Source: CAD feature listing. Evaluate the final solid. Frame: model axes, mm. A direction names the side the tool comes from. Give positions to 0.01 mm unless a question says otherwise; leave off trailing zeros. Order: outer loops, then holes, each group sorted by start corner. A loop starts at its lowest first (then second) coordinate and runs counter-clockwise, first axis right, second up. Notation, with made-up numbers: M -2,45 L 10,45 A31 cw 10,80 Z; hole C -10.5,-39.5 d10. An arc over 180 degrees is marked long. Answer in a Markdown table with one row per item. Add a question column.
(1) Section query C-C, the plane y = 8.5. Return loops of the section in (x, z), plus the area to 3 significant figures.
(2) Section query D-D, the plane x = -35. Return loops of the section in (y, z), plus the area to 3 significant figures.
(3) Mould query, pull axis Y, two halves, no side actions, for faces 1 (the face through (110.507, 6.458, 22.745)), 2 (the face through (44, 0, 0)), 3 (the face through (24, 30, 10)), 4 (the face through (-53, 0, 10)). Classes: pulls with the +Y half, pulls with the -Y half, needs draft (parallel to the pull), parting line crosses it, or undercut.
(4) Pin query (flat end, axial travel): P1, Ø5, axis at x = -48, y = -9, coming from the +Z side; P2, Ø9, axis at x = -48, y = 0, coming from the -Z side; P3, Ø1, axis at y = 16.5, z = 12, coming from the -X side; P4, Ø6.5, axis at y = -28, z = 13.5, coming from the +X side. Return the tip coordinate at first contact, or that it passes through.
(5) Material intervals for line 1 along Y through (x, z) = (0, 13); line 2 along Z through (x, y) = (-25.5, 19); line 3 along Y through (x, z) = (74.5, 28), sorted ascending.
(6) Section query B-B, the plane z = 12.5. Count the separate pieces of the cut face and the enclosed holes in it, plus the area to 3 significant figures.
(7) Section query A-A, the plane x = 0. Return loops of the section in (y, z), plus the area to 3 significant figures.
(8) Set-up query: faces 5 (the face through (90, 0, 5)), 6 (the face through (70, 9, 40)), 7 (the face through (90, -27, 10)), 8 (the face through (90, 27, 10)). Return all of +Z, -Z, +X, -X, +Y, -Y with unobstructed straight access to the full face (end or side cutting, diameter ignored); none if empty.
from build123d import *
from build123d.topology import SkipClean

# Parameters (mm, degrees)
SKETCH1_R           = 30
BOSS_EXTRUDE1_DEPTH = 20
SKETCH2_R           = 27.5
CUT_EXTRUDE1_DEPTH  = 47.904157598
BOSS_EXTRUDE2_START = -20
BOSS_EXTRUDE2_DEPTH = 20
SKETCH6_R           = 21.5
CUT_EXTRUDE2_DEPTH  = 35
SKETCH11_R          = 24
BOSS_EXTRUDE3_DEPTH = 20
BOSS_EXTRUDE4_START = -40
SKETCH12_R          = 24
BOSS_EXTRUDE4_DEPTH = 40
SKETCH13_R          = 21.5
CUT_EXTRUDE6_DEPTH  = 35
BOSS_EXTRUDE6_START = -20
BOSS_EXTRUDE6_DEPTH = 20
SKETCH15_R          = 5
CUT_EXTRUDE8_DEPTH  = 20
FILLET1_R           = 30
FILLET2_R           = 30


with BuildPart() as part:
    # Sketch1 → Boss-Extrude1 (new body)
    with BuildSketch(Plane.XY):
        Circle(SKETCH1_R)
    extrude(amount=BOSS_EXTRUDE1_DEPTH)

    # Sketch2 → Cut-Extrude1 (cut, through all)
    with BuildSketch(Plane.XY.offset(20)):
        Circle(SKETCH2_R)
    extrude(amount=-CUT_EXTRUDE1_DEPTH, mode=Mode.SUBTRACT)

    # Sketch4 → Boss-Extrude2 (add)
    with BuildSketch(Plane.XY.offset(20).offset(BOSS_EXTRUDE2_START)):
        with BuildLine():
            Line((0, 30), (90, 30))
            Line((90, 30), (90, 24))
            ThreePointArc((90, 24), (114, 0), (90, -24))
            Line((90, -24), (90, -30))
            Line((90, -30), (0, -30))
            ThreePointArc((0, -30), (30, 0), (0, 30))
        make_face()
    extrude(amount=BOSS_EXTRUDE2_DEPTH)

    # Sketch6 → Cut-Extrude2 (cut)
    with BuildSketch(Plane.XY.offset(20)):
        with Locations((90, 0)):
            Circle(SKETCH6_R)
    extrude(amount=-CUT_EXTRUDE2_DEPTH, mode=Mode.SUBTRACT)

    # Sketch11 → Boss-Extrude3 (add)
    with SkipClean():  # the faces are left unmerged after this step: merging them gives an invalid solid
        with BuildSketch(Plane.XY.offset(20)):
            with Locations((90, 0)):
                Circle(SKETCH11_R)
        extrude(amount=BOSS_EXTRUDE3_DEPTH)
    add(part.part.scale(1), mode=Mode.REPLACE)  # the faces are merged on a copy

    # Sketch12 → Boss-Extrude4 (add)
    with SkipClean():  # the faces are left unmerged after this step: merging them gives an invalid solid
        with BuildSketch(Plane.XY.offset(40).offset(BOSS_EXTRUDE4_START)):
            with Locations((90, 0)):
                Circle(SKETCH12_R)
        extrude(amount=BOSS_EXTRUDE4_DEPTH)

    # Sketch13 → Cut-Extrude6 (cut)
    with SkipClean():  # the faces are left unmerged after this step: merging them gives an invalid solid
        with BuildSketch(Plane.XY.offset(40)):
            with Locations((90, 0)):
                Circle(SKETCH13_R)
        extrude(amount=-CUT_EXTRUDE6_DEPTH, mode=Mode.SUBTRACT)

    # Sketch14 → Boss-Extrude6 (add)
    with BuildSketch(Plane.XY.offset(20).offset(BOSS_EXTRUDE6_START)):
        with BuildLine():
            ThreePointArc((0, 30), (-30, 0), (0, -30))
            Line((0, -30), (-69.770044623, -30))
            Line((-69.770044623, -30), (-69.770044623, 30))
            Line((-69.770044623, 30), (0, 30))
        make_face()
    extrude(amount=BOSS_EXTRUDE6_DEPTH)

    # Sketch15 → Cut-Extrude8 (cut)
    with BuildSketch(Plane.XY.offset(20)):
        with Locations((-48, 0)):
            Circle(SKETCH15_R)
    extrude(amount=-CUT_EXTRUDE8_DEPTH, mode=Mode.SUBTRACT)

    # Fillet1
    fillet1_edges = [part.edges().sort_by_distance(p)[0] for p in [
        (-69.770044623, -30, 10),
    ]]
    fillet(fillet1_edges, radius=FILLET1_R)

    # Fillet2
    fillet2_edges = [part.edges().sort_by_distance(p)[0] for p in [
        (-69.770044623, 30, 10),
    ]]
    fillet(fillet2_edges, radius=FILLET2_R - 0.0001)  # a hair under: the kernel refuses the full size


solid = part.part
Values follow:
| question | item | result |
|---|---|---|
| 1 | outline | M -68.54,0 L -26.15,0 L -26.15,20 L -68.54,20 Z; M 26.15,0 L 112.44,0 L 112.44,40 L 109.75,40 L 109.75,5 L 70.25,5 L 70.25,40 L 67.56,40 L 67.56,20 L 26.15,20 Z |
| 1 | area | 2,090 mm² |
| 2 | outline | M -30,0 L 30,0 L 30,20 L -30,20 Z |
| 2 | area | 1,200 mm² |
| 3 | face 1 | undercut |
| 3 | face 2 | needs draft |
| 3 | face 3 | pulls with the +Y half |
| 3 | face 4 | undercut |
| 4 | P1 | stops at z = 20 |
| 4 | P2 | passes through |
| 4 | P3 | stops at x = -65.15 |
| 4 | P4 | stops at x = 90 |
| 5 | line 1 | y = -30 to -27.5, 27.5 to 30 |
| 5 | line 2 | z = 0 to 20 |
| 5 | line 3 | y = -18.32 to -14.9, 14.9 to 18.32 |
| 6 | separate pieces | 1 |
| 6 | enclosed holes | 3 |
| 6 | area | 6,200 mm² |
| 7 | outline | M -30,0 L -27.5,0 L -27.5,20 L -30,20 Z; M 27.5,0 L 30,0 L 30,20 L 27.5,20 Z |
| 7 | area | 100 mm² |
| 8 | face 5 | +Z |
| 8 | face 6 | +Z, +X, -X, +Y, -Y |
| 8 | face 7 | +Z, -Z, +X, -Y |
| 8 | face 8 | +Z, -Z, +X, +Y |
